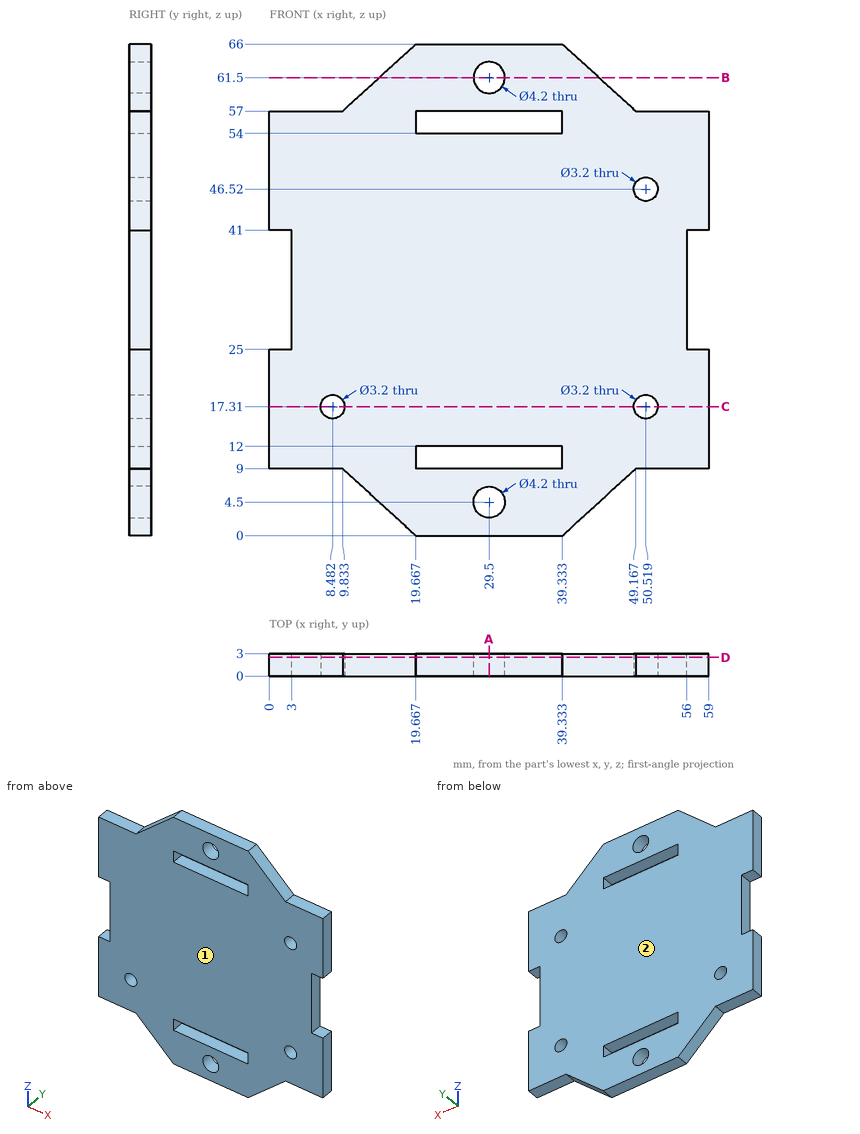
Part print with two shaded views. Sizes in mm from the minimum x, y, z corner. Round coordinates to 2 decimals unless told otherwise and drop trailing zeros. Loops run counter-clockwise (first coordinate to the right, second up) from the corner with the lowest first, then second, coordinate; pieces in that order, holes last. Notation, with made-up numbers: M 48.5,38.5 L 76.5,38.5 A33 ccw 76.5,71.5 Z; hole C 0,34.25 d5. An arc over 180 degrees is marked long. Return JSON: item names as keys, results as strings. Group by question number.
(1) Mould opens along Y. For the marked faces 1 and 2 say: +Y half, -Y half, draft (parallel to the pull), parting line (faces both ways), or undercut.
(2) Saw through at C-C, the plane z = 17.31. List the corners of the cut face in (x, y).
(3) Saw through at B-B, the plane z = 61.5. List the corners of the cut face in (x, y).
(4) Drop flat-ended pins along their axis: P1, Ø1, axis at y = 1.5, z = 31, coming from the +X side; P2, Ø1.5, axis at x = 57.5, y = 2, coming from the -Z side; P3, Ø2.5, axis at x = 29.5, z = 61.5, coming from the -Y side. Give the stop position or say it passes through.
(5) Wall check: probe 1 along X at (y, z) = (1.5, 17.31); probe 2 along X at (y, z) = (2, 56.5); probe 3 along X at (y, z) = (0.7, 4.5). Give the ranges that are in metal, low to high. Write a range as [from, to].
(6) Saw through at D-D, the plane y = 2.5. Give the number of separate pieces and of enclosed holes in the cut face, and give its area (3 significant figures).
(7) Saw through at A-A, the plane x = 29.5. List the corners of the cut face in (y, z), and give its area (3 significant figures).
Answer list:
{
 "1": {"face 1": "-Y half", "face 2": "+Y half"},
 "2": {"outline": "M 0,0 L 6.88,0 L 6.88,3 L 0,3 Z; M 10.08,0 L 48.92,0 L 48.92,3 L 10.08,3 Z; M 52.12,0 L 59,0 L 59,3 L 52.12,3 Z"},
 "3": {"outline": "M 14.75,0 L 27.4,0 L 27.4,3 L 14.75,3 Z; M 31.6,0 L 44.25,0 L 44.25,3 L 31.6,3 Z"},
 "4": {"P1": "x = 56", "P2": "z = 9", "P3": "through"},
 "5": {"probe 1": "[0, 6.88], [10.08, 48.92], [52.12, 59]", "probe 2": "[0, 19.67], [39.33, 59]", "probe 3": "[14.75, 27.4], [31.6, 44.25]"},
 "6": {"separate pieces": "1", "enclosed holes": "7", "area": "3,100 mm2"},
 "7": {"outline": "M 0,0 L 3,0 L 3,2.4 L 0,2.4 Z; M 0,6.6 L 3,6.6 L 3,9 L 0,9 Z; M 0,12 L 3,12 L 3,54 L 0,54 Z; M 0,57 L 3,57 L 3,59.4 L 0,59.4 Z; M 0,63.6 L 3,63.6 L 3,66 L 0,66 Z", "area": "155 mm2"}
}
